from build123d import *

# Parameters (mm, degrees)
SKETCH1_W           = 40
SKETCH1_H           = 40
BOSS_EXTRUDE1_DEPTH = 40
CHAMFER1_SIZE       = 5
SKETCH2_W           = 15
SKETCH2_H           = 5
BOSS_EXTRUDE2_DEPTH = 8
FILLET1_R           = 0.5
FILLET2_R           = 0.5
SKETCH3_R           = 2.5
BOSS_EXTRUDE3_DEPTH = 62


with BuildPart() as part:
    # Sketch1 → Boss-Extrude1 (new body)
    with BuildSketch(Plane.XY):
        Rectangle(SKETCH1_W, SKETCH1_H)
    extrude(amount=BOSS_EXTRUDE1_DEPTH)

    # Chamfer1
    chamfer1_edges = [part.edges().sort_by_distance(p)[0] for p in [
        (-20, 20, 20),
        (20, 20, 20),
        (20, -20, 20),
        (-20, -20, 20),
    ]]
    chamfer(chamfer1_edges, length=CHAMFER1_SIZE)

    # Sketch2 → Boss-Extrude2 (add)
    with BuildSketch(Plane.XY):
        with Locations((0, 22.5)):
            Rectangle(SKETCH2_W, SKETCH2_H)
    extrude(amount=BOSS_EXTRUDE2_DEPTH)

    # Fillet1
    fillet1_edges = [part.edges().sort_by_distance(p)[0] for p in [
        (0, -20, 0),
        (-20, 0, 0),
        (11.25, 20, 0),
        (20, 0, 0),
        (17.5, 17.5, 0),
        (-17.5, 17.5, 0),
        (17.5, -17.5, 0),
        (-17.5, -17.5, 0),
        (-11.25, 20, 0),
        (-7.5, 22.5, 0),
        (7.5, 22.5, 0),
        (0, 25, 0),
    ]]
    fillet(fillet1_edges, radius=FILLET1_R)

    # Fillet2
    # the kernel refuses this fillet: 0.5 mm, written as the material it takes off along each edge
    with BuildSketch(Plane(origin=(-7, 24.5, 0.5), x_dir=(0, 1, 0), z_dir=(-1, 0, 0))) as fillet2_piece_1_section:
        Polygon((0, 0), (FILLET2_R, 0), (FILLET2_R, FILLET2_R), (0, FILLET2_R), align=None)
    fillet2_piece_1 = extrude(amount=FILLET2_R, mode=Mode.PRIVATE)
    fillet2_piece_1 = fillet2_piece_1 - Plane(origin=(-7, 24.5, 0.5), x_dir=(0, -0.7071067811865475, 0.7071067811865475), z_dir=(-1, 0, 0)) * Sphere(FILLET2_R, mode=Mode.PRIVATE)
    add(fillet2_piece_1, mode=Mode.SUBTRACT)
    with BuildSketch(Plane(origin=(7, 24.5, 0.5), x_dir=(0, 1, 0), z_dir=(1, 0, 0))) as fillet2_piece_2_section:
        Polygon((0, 0), (FILLET2_R, 0), (FILLET2_R, -FILLET2_R), (0, -FILLET2_R), align=None)
    fillet2_piece_2 = extrude(amount=FILLET2_R, mode=Mode.PRIVATE)
    fillet2_piece_2 = fillet2_piece_2 - Plane(origin=(7, 24.5, 0.5), x_dir=(0, -0.7071067811865475, 0.7071067811865475), z_dir=(1, 0, 0)) * Sphere(FILLET2_R, mode=Mode.PRIVATE)
    add(fillet2_piece_2, mode=Mode.SUBTRACT)
    with BuildSketch(Plane(origin=(-7.5, 25, 0.5), x_dir=(0, -1, 0), z_dir=(0, 0, 1))) as fillet2_piece_3:
        with BuildLine():
            CenterArc((FILLET2_R, FILLET2_R), FILLET2_R, 180, 90)
            Line((0, FILLET2_R), (0, 0))
            Line((0, 0), (FILLET2_R, 0))
        make_face()
    extrude(amount=8.75, mode=Mode.SUBTRACT)
    with BuildSketch(Plane(origin=(7.5, 25, 0.5), x_dir=(0, -1, 0), z_dir=(0, 0, 1))) as fillet2_piece_4:
        with BuildLine():
            CenterArc((FILLET2_R, -FILLET2_R), FILLET2_R, 90, 90)
            Line((0, -FILLET2_R), (0, 0))
            Line((0, 0), (FILLET2_R, 0))
        make_face()
    extrude(amount=8.75, mode=Mode.SUBTRACT)

    # Sketch3 → Boss-Extrude3 (add)
    with BuildSketch(Plane.XY):
        Circle(SKETCH3_R)
    extrude(amount=BOSS_EXTRUDE3_DEPTH)


solid = part.part
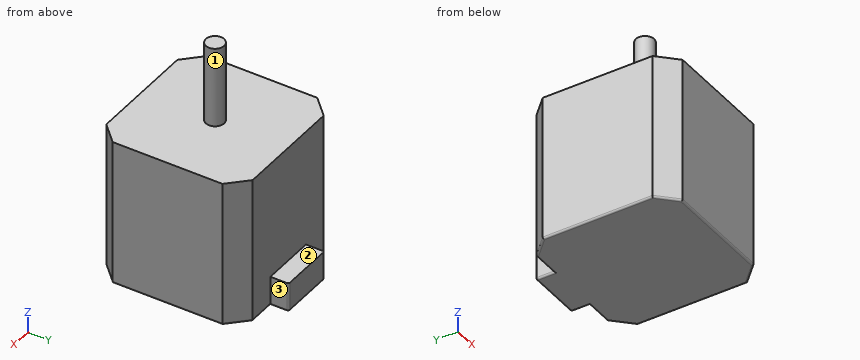
Model file for the job. Use its own axes, mm. Face numbers are marked on the shaded views. A direction names the side the tool comes from. Give positions to 0.01 mm unless a question says otherwise; leave off trailing zeros. Order: outer loops, then holes, each group sorted by start corner. A loop starts at its lowest first (then second) coordinate and runs counter-clockwise, first axis right, second up. Notation, with made-up numbers: (-29, -34.75) - (7, -34.75) arc R26 ccw to (7, 1.25) - close; hole circle Ø11 at (9.25, -40). An arc over 180 degrees is marked (long way). Write item = value, one per line. Start each with the question number.
1. Cut at A-A, the plane z = 25. List the corners of the cut face in (x, y), and give its area (3 significant figures).
2. Cut at B-B, the plane y = 0. List the corners of the cut face in (x, z).
3. Drop flat-ended pins along their axis: P1, Ø1.5, axis at x = 2.5, y = 22, coming from the +Z side; P2, Ø12, axis at x = -1, y = 5.5, coming from the +Z side; P3, Ø1.3, axis at y = 21.5, z = 6, coming from the +X side; P4, Ø4, axis at x = -6, z = 10.5, coming from the +Y side. Give the stop position or say it passes through.
4. Cut at C-C, the plane x = 0. List the corners of the cut face in (y, z), and give its area (3 significant figures).
5. Probe line 1 along Z through (x, y) = (16, 7); line 2 along Y through (x, z) = (-13, 36.5); line 3 along X through (y, z) = (17, 33.5). List the from-to ranges inside material, lowest first.
6. Cut at D-D, the plane y = 7.5. List the corners of the cut face in (x, z).
7. Which spindle directions (+Z, -Z, +X, -X, +Y, -Y) get a long thin tool onto all of the face, cutting with end or side? Do the marked faces 1, 2 and 3. Say none if no direction does.
Taken from the geometry:
q1.outline = (-20, -15) - (-15, -20) - (15, -20) - (20, -15) - (20, 15) - (15, 20) - (-15, 20) - (-20, 15) - close
q1.area = 1,550 mm²
q2.outline = (-20, 0.5) arc R0.5 ccw to (-19.5, 0) - (19.5, 0) arc R0.5 ccw to (20, 0.5) - (20, 40) - (2.5, 40) - (2.5, 62) - (-2.5, 62) - (-2.5, 40) - (-20, 40) - close
q3.P1 = 8
q3.P2 = 62
q3.P3 = 7.5
q3.P4 = 20
q4.outline = (-20, 0.5) arc R0.5 ccw to (-19.5, 0) - (24.5, 0) arc R0.5 ccw to (25, 0.5) - (25, 8) - (20, 8) - (20, 40) - (2.5, 40) - (2.5, 62) - (-2.5, 62) - (-2.5, 40) - (-20, 40) - close
q4.area = 1,750 mm²
q5.line_1 = 0 to 40
q5.line_2 = -20 to 20
q5.line_3 = -18 to 18
q6.outline = (-20, 0.5) arc R0.5 ccw to (-19.5, 0) - (19.5, 0) arc R0.5 ccw to (20, 0.5) - (20, 40) - (-20, 40) - close
q7.face_1 = +Z
q7.face_2 = +Z, +X, -X, +Y
q7.face_3 = +Z, -Z, +X, +Y
